Geometry: final body of the model. Coordinates: model frame, mm. A direction names the side the tool comes from. Give positions to 0.01 mm unless a question says otherwise; leave off trailing zeros. Write each loop counter-clockwise with the first axis right and the second up, starting at its lowest first coordinate (ties: lowest second). Pieces come first, ordered by that corner, then holes.
Q1. Section A-A (x = -158.75). Return the cut outline in (y, z).
Q2. Line query: line 1 (Z direction, x = -158.75, y = 210.5); line 2 (Z direction, x = -158, y = 213); line 3 (X direction, y = 211.75, z = -19.05). Output: solid intervals per line, ascending.
Q3. Mould query, pull axis X, two halves, no side actions, for faces 1 (the cylindrical face through (-174.1, 200.1, 0.5)), 2 (the cylindrical face through (-162.237, 211.202, -18.276)), 3 (the conical face through (-190.72, 168.95, 0.4)). Classes: +X half, -X half, draft (parallel to the pull), parting line (faces both ways), or undercut.
Q4. Reachability of faces 4 (the flat face through (-175, 201, -37.665)), 5 (the cylindrical face through (-183.625, 203.277, 0.531)) from +Z, -Z, +X, -X, +Y, -Y: full face, straight path, thin tool, end or side. Return the list, or none.
Q5. Pin query (flat end, axial travel): pin 1 Ø2 at (y, z) = (185.5, 1.5) entering from -X; pin 2 Ø25 at (x, z) = (-156.5, 15) entering from -Y; pin 3 Ø6.5 at (x, z) = (-158.75, 19.05) entering from +Y; pin 4 Ø12 at (x, z) = (-190, -24) entering from -Y. Return the tip coordinate at first contact, or that it passes through.
from build123d import *

# Parameters (mm, degrees)
REVOLVE1_ANGLE          = 30
FILLET1_R               = 7.5
CUT_EXTRUDE1_DEPTH      = 207.295163461
CUT_EXTRUDE1_DEPTH_BACK = 207.295163461
SKETCH3_R               = 3.571875
SKETCH4_OUTSIDE_W       = 82.664
SKETCH4_OUTSIDE_H       = 128.62
SKETCH4_OUTSIDE_W_2     = 74.859969382
SKETCH4_OUTSIDE_H_2     = 75.329921726
CUT_EXTRUDE2_DEPTH      = 209.298230862
FILLET2_R               = 10


with BuildPart() as part:
    # Sketch2 → Revolve1 (revolve, symmetric)
    with BuildSketch(Plane.XY) as revolve1_sk:
        with BuildLine():
            Line((-196.144484664, 171.227986779), (-187.361895799, 167.541286653))
            ThreePointArc((-187.361895799, 167.541286653), (-181.203221282, 180.846197706), (-174.101233777, 193.672409282))
            Line((-174.101233777, 193.672409282), (-174.101233777, 206.372409282))
            Line((-174.101233777, 206.372409282), (-145.526233777, 206.372409282))
            Line((-145.526233777, 206.372409282), (-145.526233777, 215.897409282))
            Line((-145.526233777, 215.897409282), (-183.626233777, 215.897409282))
            Line((-183.626233777, 215.897409282), (-183.626233777, 196.285035224))
            ThreePointArc((-183.626233777, 196.285035224), (-190.298222707, 183.962773472), (-196.144484664, 171.227986779))
        make_face()
    revolve(axis=Axis((0, 0, 0), (0, 1, 0)), revolution_arc=REVOLVE1_ANGLE / 2)
    revolve(revolve1_sk.sketch, axis=Axis((0, 0, 0), (0, -1, 0)), revolution_arc=REVOLVE1_ANGLE / 2)

    # Fillet1
    fillet1_edges = [part.edges().sort_by_distance(p)[0] for p in [
        (-183.626233777, 196.285035224, 0),
        (-183.626233777, 215.897409282, 0),
    ]]
    fillet(fillet1_edges, radius=FILLET1_R)

    # Sketch3 → Cut-Extrude1 (cut, two sides: drawn at the far end of the back side and taken through both)
    with BuildSketch(Plane.XZ.offset(-206.372409282).offset(-CUT_EXTRUDE1_DEPTH_BACK)):
        with Locations(Location((-158.75, 19.05, 0), (0, 0, 270))):
            Circle(SKETCH3_R)
        with Locations(Location((-158.75, -19.05, 0), (0, 0, 270))):
            Circle(SKETCH3_R)
    extrude(amount=CUT_EXTRUDE1_DEPTH + CUT_EXTRUDE1_DEPTH_BACK, mode=Mode.SUBTRACT)

    # Sketch4 outside → Cut-Extrude2 (cut, through all)
    with BuildSketch(Plane(origin=(0, 215.897409282, 0), x_dir=(1, 0, 0), z_dir=(0, 1, 0))):
        with Locations((-168.356, 0)):
            Rectangle(SKETCH4_OUTSIDE_W, SKETCH4_OUTSIDE_H)
        with Locations((-177.997532298, 0)):
            Rectangle(SKETCH4_OUTSIDE_W_2, SKETCH4_OUTSIDE_H_2, mode=Mode.SUBTRACT)
    extrude(amount=-CUT_EXTRUDE2_DEPTH, mode=Mode.SUBTRACT)

    # Fillet2
    fillet2_edges = [part.edges().sort_by_distance(p)[0] for p in [
        (-140.567547607, 211.134909282, 37.664960863),
        (-188.015889107, 169.383911967, 37.664960863),
        (-188.015889107, 169.383911967, -37.664960863),
        (-140.567547607, 211.134909282, -37.664960863),
    ]]
    fillet(fillet2_edges, radius=FILLET2_R)


solid = part.part
Computed:
1. outline: (206.37, -37.66) - (215.9, -37.66) - (215.9, -22.62) - (206.37, -22.62) - close; (206.37, -15.48) - (215.9, -15.48) - (215.9, 15.48) - (206.37, 15.48) - close; (206.37, 22.62) - (215.9, 22.62) - (215.9, 37.66) - (206.37, 37.66) - close
2. line 1: z = -37.66 to -22.62, -15.48 to 15.48, 22.62 to 37.66
2. line 2: z = -37.66 to -22.54, -15.56 to 15.56, 22.54 to 37.66
2. line 3: x = -181.84 to -162.32, -155.18 to -144.27
3. face 1: +X half
3. face 2: undercut
3. face 3: -X half
4. face 4: -Z, +X, -X, +Y, -Y
4. face 5: -X, +Y
5. pin 1: stops at x = -190.02
5. pin 2: stops at y = 206.37
5. pin 3: passes through
5. pin 4: stops at y = 167.54
